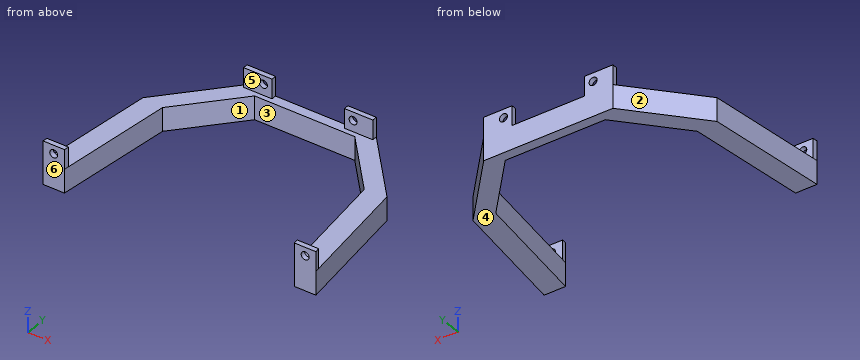
from build123d import *

# Parameters (mm, degrees)
BOSS_EXTRUDE1_DEPTH      = 10
BOSS_EXTRUDE1_DEPTH_BACK = 2.055125775
BOSS_EXTRUDE2_DEPTH      = 10
SKETCH3_R                = 2.05
CUT_EXTRUDE1_DEPTH       = 10
SKETCH4_W                = 14.568281885
SKETCH4_H                = 2.5
BOSS_EXTRUDE3_DEPTH      = 10
SKETCH6_R                = 2.05
CUT_EXTRUDE2_DEPTH       = 10


with BuildPart() as part:
    # Sketch1 → Boss-Extrude1 (new, two sides: drawn at the far end of the back side and taken through both)
    with BuildSketch(Plane.XY.offset(-BOSS_EXTRUDE1_DEPTH_BACK)):
        Polygon((0, 0), (-11, 0), (-3.916610397, 61.857854845), (25.860231814, 95), (92.139768186, 95), (121.30603718, 61.857854845), (129, 0), (118, 0), (110.448917943, 60.709123335), (84.671902488, 90), (33.26848477, 90), (6.951847491, 60.709123335), align=None)
    extrude(amount=BOSS_EXTRUDE1_DEPTH + BOSS_EXTRUDE1_DEPTH_BACK)

    # Sketch2 → Boss-Extrude2 (add)
    with BuildSketch(Plane.XY.offset(10)):
        Polygon((-11, 0), (0, 0), (0.286276885, 2.5), (-10.713723115, 2.5), align=None)
        Polygon((118, 0), (129, 0), (128.689046652, 2.5), (117.689046652, 2.5), align=None)
    extrude(amount=BOSS_EXTRUDE2_DEPTH)

    # Sketch3 → Cut-Extrude1 (cut)
    with BuildSketch(Plane(origin=(0, 2.5, 0), x_dir=(1, 0, 0), z_dir=(0, 1, 0))):
        with Locations(Location((-5.5, -15.687372709, 0), (0, 0, 180))):
            Circle(SKETCH3_R)
        with Locations(Location((123.5, -15.687372709, 0), (0, 0, 180))):
            Circle(SKETCH3_R)
    extrude(amount=-CUT_EXTRUDE1_DEPTH, mode=Mode.SUBTRACT)

    # Sketch4 → Boss-Extrude3 (add)
    with BuildSketch(Plane.XY.offset(10)):
        with Locations((33.144372757, 93.75)):
            Rectangle(SKETCH4_W, SKETCH4_H)
        with Locations((84.855627244, 93.75)):
            Rectangle(SKETCH4_W, SKETCH4_H)
    extrude(amount=BOSS_EXTRUDE3_DEPTH)

    # Sketch6 → Cut-Extrude2 (cut)
    with BuildSketch(Plane(origin=(0, 95, 0), x_dir=(1, 0, 0), z_dir=(0, 1, 0))):
        with Locations(Location((36, -15.687372709, 0), (0, 0, 270))):
            Circle(SKETCH6_R)
        with Locations(Location((82, -15.687372709, 0), (0, 0, 270))):
            Circle(SKETCH6_R)
    extrude(amount=-CUT_EXTRUDE2_DEPTH, mode=Mode.SUBTRACT)


solid = part.part
Read the model definition and answer for the solid it produces. Units are mm, in the model's axes. Face numbers are marked on the shaded views. A direction names the side the tool comes from. Round coordinates to 2 decimals unless told otherwise and drop trailing zeros. Order: outer loops, then holes, each group sorted by start corner. A loop starts at its lowest first (then second) coordinate and runs counter-clockwise, first axis right, second up.
1) The part is cut by section C-C on y = 21.5. Write down the section's boundary in (x, z).
2) Flat-ended cylindrical pins translate along their axes: pin 1 (3 mm diameter, centred on y = 94.5, z = 12.5, fed in from +X); pin 2 (5 mm diameter, centred on x = 126, z = 17.5, fed in from +Y); pin 3 (5 mm diameter, centred on x = 86.5, z = 15, fed in from -Y); pin 4 (8 mm diameter, centred on y = 78.5, z = 17.5, fed in from -X). Find the tip coordinate at first contact, or state that the pin passes through.
3) The part is cut by section A-A on z = 11.75. Write down the section's boundary in (x, y), plus the area to 3 significant figures.
4) The mould has two halves that part along X. Classify the marked faces 1, 2, 3 and 4: released by +X, released by -X, zero draft, split by the parting line, or undercut.
5) For the marked faces 5 and 6, determine the directions among +Z, -Z, +X, -X, +Y, -Y from which every point of the face is accessible in a straight line to the end or side of a thin tool.
6) The part is cut by section D-D on z = 3.75. Write down the section's boundary in (x, y), plus the area to 3 significant figures.
7) Straight lines are drawn through the part: L1, parallel to Z at x = 123.5, y = 1.95; L2, parallel to Y at x = 75, z = 2.5; L3, parallel to X at y = 79, z = 0.5. For each, find the intervals that lie inside material, in ascending order.
8) The part is cut by section B-B on x = 82. Write down the section's boundary in (y, z).
Resolved:
1. outline: (-8.54, -2.06) - (2.46, -2.06) - (2.46, 10) - (-8.54, 10) - close; (115.33, -2.06) - (126.33, -2.06) - (126.33, 10) - (115.33, 10) - close
2. pin 1: stops at x = 92.14
2. pin 2: stops at y = 2.5
2. pin 3: stops at y = 92.5
2. pin 4: passes through
3. outline: (-11, 0) - (0, 0) - (0.29, 2.5) - (-10.71, 2.5) - close; (25.86, 92.5) - (40.43, 92.5) - (40.43, 95) - (25.86, 95) - close; (77.57, 92.5) - (92.14, 92.5) - (92.14, 95) - (77.57, 95) - close; (117.69, 2.5) - (118, 0) - (129, 0) - (128.69, 2.5) - close
3. area: 128 mm2
4. face 1: undercut
4. face 2: released by -X
4. face 3: undercut
4. face 4: zero draft
5. face 5: +Z, +X, -X, -Y
5. face 6: +Z, -Z, +X, -X, -Y
6. outline: (-11, 0) - (0, 0) - (6.95, 60.71) - (33.27, 90) - (84.67, 90) - (110.45, 60.71) - (118, 0) - (129, 0) - (121.31, 61.86) - (92.14, 95) - (25.86, 95) - (-3.92, 61.86) - close
6. area: 2,380 mm2
7. L1: z = -2.06 to 13.64, 17.74 to 20
7. L2: y = 90 to 95
7. L3: x = 11.48 to 23.39, 94.35 to 106.22
8. outline: (90, -2.06) - (95, -2.06) - (95, 13.64) - (92.5, 13.64) - (92.5, 10) - (90, 10) - close; (92.5, 17.74) - (95, 17.74) - (95, 20) - (92.5, 20) - close
